Check sheet for the modelled part. Datum: model origin and axes. Units: mm. A direction names the side the tool comes from. Round coordinates to 2 decimals unless told otherwise and drop trailing zeros. Order: outer loops, then holes, each group sorted by start corner. A loop starts at its lowest first (then second) coordinate and runs counter-clockwise, first axis right, second up.
```python
from build123d import *
from OCP.BRepFilletAPI import BRepFilletAPI_MakeChamfer

# Parameters (mm, degrees)
BOSS_EXTRU_1_DEPTH           = 3.8
BOSS_EXTRU_1_TAPER           = 45
COQUE2_DEPTH                 = 1.8
COQUE2_DRAFT                 = 45
CHANFREIN1_SIZE              = 1
CHANFREIN1_SIZE2             = 0.707106781
ENL_V_MAT_EXTRU_1_REACH      = 39.355
ESQUISSE2_R                  = 1.5
ENL_V_MAT_EXTRU_2_REACH      = 39.215
ESQUISSE3_R                  = 1.55
ESQUISSE3_R_2                = 2
ESQUISSE4_W                  = 4.3
ESQUISSE4_H                  = 4.3
BOSS_EXTRU_2_DEPTH           = 3
CHANFREIN2_SIZE              = 1
CHANFREIN2_OF_SYM_TRIE1_SIZE = 1


# Read off the part's stored shape, not the designer's step: Coque2
with BuildPart() as part:
    # Esquisse1 → Boss.-Extru.1 (new body)
    with BuildSketch(Plane(origin=(0, 0, 0), x_dir=(1, 0, 0), z_dir=(0, 1, 0))):
        with BuildLine():
            ThreePointArc((-20, 14.8), (-34.8, 0), (-20, -14.8))
            Line((-20, -14.8), (20, -14.8))
            ThreePointArc((20, -14.8), (34.8, 0), (20, 14.8))
            Line((20, 14.8), (-20, 14.8))
        make_face()
    extrude(amount=BOSS_EXTRU_1_DEPTH, taper=BOSS_EXTRU_1_TAPER)


with BuildPart() as coque2_tool:
    # Coque2 outline → Coque2 (with draft: the straight prism first)
    with BuildSketch(Plane(origin=(0, 1.8, 0), x_dir=(1, 0, 0), z_dir=(0, 1, 0))):
        with BuildLine():
            Line((-20, -10.171572875), (20, -10.171572875))
            ThreePointArc((20, -10.171572875), (30.171572875, 0), (20, 10.171572875))
            Line((20, 10.171572875), (-20, 10.171572875))
            ThreePointArc((-20, 10.171572875), (-30.171572875, 0), (-20, -10.171572875))
        make_face()
    extrude(amount=-COQUE2_DEPTH)
    # Coque2: the draft: its side faces are tilted about the plane it starts from
    coque2_sides = [coque2_tool.faces().sort_by_distance(p)[0] for p in [
        (0, 0.9, 10.171572875),
        (30.171572875, 0.9, 0),
        (0, 0.9, -10.171572875),
        (-30.171572875, 0.9, 0),
    ]]
    draft(coque2_sides, Plane(origin=(0, 1.8, 0), x_dir=(1, 0, 0), z_dir=(0, 1, 0)), COQUE2_DRAFT)


with BuildPart() as part_1:
    add(part.part)

    # Coque2: cut by coque2_tool
    add(coque2_tool.part, mode=Mode.SUBTRACT)

    # Chanfrein1: one chamfer whose edges measure the first distance from different faces: ONE call of the kernel's chamfer builder (chamfer() names one face for all edges)
    chanfrein1_edges_1 = [part_1.edges().sort_by_distance(p)[0] for p in [
        (0, 0, -14.8),
        (0, 0, 14.8),
        (-34.8, 0, 0),
    ]]
    chanfrein1_side_1 = [part_1.faces().sort_by_distance(p)[0] for p in [
        (0, 0, -14.043672029),
    ]]
    chanfrein1_edges_2 = [part_1.edges().sort_by_distance(p)[0] for p in [
        (34.8, 0, 0),
    ]]
    chanfrein1_side_2 = [part_1.faces().sort_by_distance(p)[0] for p in [
        (32.9, 1.9, 0),
    ]]
    chanfrein1 = BRepFilletAPI_MakeChamfer(part_1.part.solid().wrapped)
    for e in chanfrein1_edges_1:
        chanfrein1.Add(CHANFREIN1_SIZE, CHANFREIN1_SIZE2, e.wrapped, chanfrein1_side_1[0].wrapped)  # the first distance lies on this face
    for e in chanfrein1_edges_2:
        chanfrein1.Add(CHANFREIN1_SIZE, CHANFREIN1_SIZE2, e.wrapped, chanfrein1_side_2[0].wrapped)  # the first distance lies on this face
    add(Compound.cast(chanfrein1.Shape()), mode=Mode.REPLACE)

    # Esquisse2 → Enlèv. mat.-Extru.1 (cut, up to next)
    with BuildSketch(Plane(origin=(0, 3.8, 0), x_dir=(1, 0, 0), z_dir=(0, 1, 0)), mode=Mode.PRIVATE) as enl_v_mat_extru_1_sk1:
        with Locations(Location((-28, 0, 0), (0, 0, 270))):
            Circle(ESQUISSE2_R)
    enl_v_mat_extru_1_tool1 = extrude(enl_v_mat_extru_1_sk1.sketch, amount=-ENL_V_MAT_EXTRU_1_REACH, mode=Mode.PRIVATE) & part_1.part
    # Esquisse2 → Enlèv. mat.-Extru.1 (cut, up to next)
    with BuildSketch(Plane(origin=(0, 3.8, 0), x_dir=(1, 0, 0), z_dir=(0, 1, 0)), mode=Mode.PRIVATE) as enl_v_mat_extru_1_sk2:
        with Locations(Location((28, 0, 0), (0, 0, 270))):
            Circle(ESQUISSE2_R)
    enl_v_mat_extru_1_tool2 = extrude(enl_v_mat_extru_1_sk2.sketch, amount=-ENL_V_MAT_EXTRU_1_REACH, mode=Mode.PRIVATE) & part_1.part
    add(enl_v_mat_extru_1_tool1.solids().sort_by_distance((-28, 3.8, 0))[0], mode=Mode.SUBTRACT)
    add(enl_v_mat_extru_1_tool2.solids().sort_by_distance((28, 3.8, 0))[0], mode=Mode.SUBTRACT)

    # Esquisse3 → Enlèv. mat.-Extru.2 (cut, up to next)
    with BuildSketch(Plane.XZ.offset(-1.8), mode=Mode.PRIVATE) as enl_v_mat_extru_2_sk1:
        with Locations(Location((0, -5, 0), (0, 0, 270))):
            Circle(ESQUISSE3_R)
    enl_v_mat_extru_2_tool1 = extrude(enl_v_mat_extru_2_sk1.sketch, amount=-ENL_V_MAT_EXTRU_2_REACH, mode=Mode.PRIVATE) & part_1.part
    # Esquisse3 → Enlèv. mat.-Extru.2 (cut, up to next)
    with BuildSketch(Plane.XZ.offset(-1.8), mode=Mode.PRIVATE) as enl_v_mat_extru_2_sk2:
        with Locations(Location((10, 5, 0), (0, 0, 270))):
            Circle(ESQUISSE3_R_2)
    enl_v_mat_extru_2_tool2 = extrude(enl_v_mat_extru_2_sk2.sketch, amount=-ENL_V_MAT_EXTRU_2_REACH, mode=Mode.PRIVATE) & part_1.part
    # Esquisse3 → Enlèv. mat.-Extru.2 (cut, up to next)
    with BuildSketch(Plane.XZ.offset(-1.8), mode=Mode.PRIVATE) as enl_v_mat_extru_2_sk3:
        with Locations(Location((0, 5, 0), (0, 0, 270))):
            Circle(ESQUISSE3_R_2)
    enl_v_mat_extru_2_tool3 = extrude(enl_v_mat_extru_2_sk3.sketch, amount=-ENL_V_MAT_EXTRU_2_REACH, mode=Mode.PRIVATE) & part_1.part
    # Esquisse3 → Enlèv. mat.-Extru.2 (cut, up to next)
    with BuildSketch(Plane.XZ.offset(-1.8), mode=Mode.PRIVATE) as enl_v_mat_extru_2_sk4:
        with Locations(Location((-10, 5, 0), (0, 0, 270))):
            Circle(ESQUISSE3_R_2)
    enl_v_mat_extru_2_tool4 = extrude(enl_v_mat_extru_2_sk4.sketch, amount=-ENL_V_MAT_EXTRU_2_REACH, mode=Mode.PRIVATE) & part_1.part
    add(enl_v_mat_extru_2_tool1.solids().sort_by_distance((0, 1.8, -5))[0], mode=Mode.SUBTRACT)
    add(enl_v_mat_extru_2_tool2.solids().sort_by_distance((10, 1.8, 5))[0], mode=Mode.SUBTRACT)
    add(enl_v_mat_extru_2_tool3.solids().sort_by_distance((0, 1.8, 5))[0], mode=Mode.SUBTRACT)
    add(enl_v_mat_extru_2_tool4.solids().sort_by_distance((-10, 1.8, 5))[0], mode=Mode.SUBTRACT)

    # Esquisse4 → Boss.-Extru.2 (add)
    with BuildSketch(Plane.ZY.offset(-20)):
        Polygon((9, 3.8), (1, 3.8), (1, 14.1), (5, 14.1), (9, 14.1), align=None)
        with Locations((5, 9.95)):
            Rectangle(ESQUISSE4_W, ESQUISSE4_H, mode=Mode.SUBTRACT)
    boss_extru_2 = extrude(amount=BOSS_EXTRU_2_DEPTH)

    # Chanfrein2
    chanfrein2_edges = [part_1.edges().sort_by_distance(p)[0] for p in [
        (18.5, 14.1, 9),
        (18.5, 14.1, 1),
    ]]
    chamfer(chanfrein2_edges, length=CHANFREIN2_SIZE)

    # Symétrie1: Boss.-Extru.2 across plane
    add(boss_extru_2.mirror(Plane(origin=(0, 0, 0), x_dir=(0, 0, 1), z_dir=(1, 0, 0))))

    # Chanfrein2 of Symétrie1
    chanfrein2_of_sym_trie1_edges = [part_1.edges().sort_by_distance(p)[0] for p in [
        (-18.5, 14.1, 9),
        (-18.5, 14.1, 1),
    ]]
    chamfer(chanfrein2_of_sym_trie1_edges, length=CHANFREIN2_OF_SYM_TRIE1_SIZE)


solid = part_1.part
```
Item 1: Scan lines: line 1 along X through (y, z) = (3.3, 5); line 2 along X through (y, z) = (13, 7.25); line 3 along X through (y, z) = (2.35, 0). Record each from-to range of solid material in increasing order.
Answer:
line 1: x = -30.36 to -12, -8 to -2, 2 to 8, 12 to 30.36
line 2: x = -20 to -17, 17 to 20
line 3: x = -32.45 to -29.5, -26.5 to 26.5, 29.5 to 32.45
Item 2: Sectioned sample at B-B (y = 5). Record the cut outline in (x, z), and give its area (3 significant figures).
Answer:
outline: (-20, 1) - (-17, 1) - (-17, 9) - (-20, 9) - close; (17, 1) - (20, 1) - (20, 9) - (17, 9) - close
area: 48.0 mm2
Item 3: Go/stop test with flat-tipped pins: P1, Ø6, axis at x = -24.5, y = 6, coming from the -Z side; P2, Ø4.5, axis at x = 10, z = 5, coming from the +Y side; P3, Ø3.5, axis at x = -19, y = 9.5, coming from the +Z side. Record where each tip stops, or that it passes through.
Answer:
P1: stops at z = -11.09
P2: stops at y = 3.8
P3: stops at z = 9
Item 4: Release check for a two-part mould opening along Z. For faces 1 (the conical face through (30.46, 1.51, 0.23)), 2 (the conical face through (31.2, 3.6, 0.2)), 3 (the flat face through (-19, 9, 9)), 4 (the flat face through (-0.2, 0, 12.3)) record: released by +Z, released by -Z, zero draft, split by the parting line, or undercut.
Answer:
face 1: undercut
face 2: split by the parting line
face 3: released by +Z
face 4: zero draft
Item 5: Sectioned sample at C-C (z = 0). Record the cut outline in (x, y), and give its area (3 significant figures).
Answer:
outline: (-34.3, 0.5) - (-33.8, 0) - (-31.97, 0) - (-30.17, 1.8) - (-29.5, 1.8) - (-29.5, 3.8) - (-31, 3.8) - close; (-26.5, 1.8) - (26.5, 1.8) - (26.5, 3.8) - (-26.5, 3.8) - close; (29.5, 1.8) - (30.17, 1.8) - (31.97, 0) - (33.8, 0) - (34.3, 0.5) - (31, 3.8) - (29.5, 3.8) - close
area: 126 mm2
Item 6: Sectioned sample at D-D (x = -19). Record the cut outline in (y, z).
Answer:
outline: (0, -13.8) - (0.5, -14.3) - (3.8, -11) - (3.8, 1) - (13.1, 1) - (14.1, 2) - (14.1, 8) - (13.1, 9) - (3.8, 9) - (3.8, 11) - (0.5, 14.3) - (0, 13.8) - (0, 11.97) - (1.8, 10.17) - (1.8, -10.17) - (0, -11.97) - close; hole (7.8, 2.85) - (12.1, 2.85) - (12.1, 7.15) - (7.8, 7.15) - close
Item 7: Sectioned sample at A-A (x = -10). Record the cut outline in (y, z), and give its area (3 significant figures).
Answer:
outline: (0, -13.8) - (0.5, -14.3) - (3.8, -11) - (3.8, 3) - (1.8, 3) - (1.8, -10.17) - (0, -11.97) - close; (0, 11.97) - (1.8, 10.17) - (1.8, 7) - (3.8, 7) - (3.8, 11) - (0.5, 14.3) - (0, 13.8) - close
area: 49.7 mm2
Item 8: Access from +Z, -Z, +X, -X, +Y, -Y to the whole of each face (thin tool, end or side, straight path). Record for faces 5 (the flat face through (-17, 7, 5)), 6 (the flat face through (-20, 7, 5)), 7 (the flat face through (-19, 7.8, 5)), 8 (the flat face through (20, 7, 5)), 9 (the flat face through (0, 1.8, 0)).
Answer:
face 5: +Z, -Z, +Y
face 6: +Z, -Z, -X, +Y
face 7: +X, -X
face 8: +Z, -Z, +X, +Y
face 9: -Y
